The listing builds one solid part. Answer for the finished solid, in the listing's coordinates (mm). Coordinates: 2 decimals unless noted, no trailing zeros. Write each loop counter-clockwise with the first axis right and the second up, starting at its lowest first coordinate (ties: lowest second). Pieces come first, ordered by that corner, then holes.
from build123d import *

# Parameters (mm, degrees)
F2_SIZE2 = 0.21996
F2_SIZE  = 0.12699


# Not quite as in the source:
# - a fillet or chamfer is up to 0.001 mm smaller than in the source, because OpenCascade refuses the exact size


with BuildPart() as f1:
    # F0 (on Front) → F1 (revolve)
    with BuildSketch(Plane.XZ):
        Polygon((-38.1, 9.779), (0, 9.779), (0, 10.033), (-3.81, 10.033), (-3.81, 10.795), (-38.1, 10.795), align=None)
    revolve(axis=Axis((-19.05, 0, 0), (-1, 0, 0)))

    # F2 (size 0.127 and 0.2199704526 in the source; OpenCascade refuses exactly that, so slightly less here)
    f2_edges = [f1.edges().sort_by_distance(p)[0] for p in [
        (0, 0, -10.033),
        (0, 0, -9.779),
    ]]
    f2_side = f1.faces().sort_by_distance((0, 0, -9.807378))[0]
    chamfer(f2_edges, length=F2_SIZE, length2=F2_SIZE2, reference=f2_side)


solid = f1.part
Q1. Find the intervals of material crossed by probe 1 along Y at (x, z) = (-7.5, 0) (3 decimals); probe 2 along Z at (x, y) = (-5, -1); probe 3 along Z at (x, y) = (-15, 5), in increasing order.
Answers below:
probe 1: y = -10.795 to -9.779, 9.779 to 10.795
probe 2: z = -10.75 to -9.73, 9.73 to 10.75
probe 3: z = -9.57 to -8.4, 8.4 to 9.57
Q2. The part is cut by section C-C, the plane x = -11. Write down the section's boundary in (y, z) (3 decimals), then the cut area to 3 significant figures.
Answers below:
outline: circle Ø21.59 at (0, 0); hole circle Ø19.558 at (0, 0)
area: 65.7 mm2
Q3. Given pin 1 (1.5 mm diameter, centred on x = -33, z = 7, fed in from +Y); pin 2 (11 mm diameter, centred on y = 4, z = -3.5, fed in from +X); pin 3 (1.5 mm diameter, centred on x = -25, z = -2.5, fed in from -Y); pin 4 (3 mm diameter, centred on x = -19.5, y = 7, fed in from -Z), each flat-ended and moving along its own axis, determine where each tip first touches the part or whether it passes through.
Answers below:
pin 1: stops at y = 8.8
pin 2: stops at x = 0
pin 3: stops at y = -10.65
pin 4: stops at z = -9.29
Q4. Determine the mould class of faces 1 (the face through (-18.895, -9.546, -2.12)), 2 (the face through (-3.81, -10, -3)), 3 (the face through (-2.04, -9.794, -2.175)) for opening direction Z: released by +Z, released by -Z, zero draft, split by the parting line, or undercut.
Answers below:
face 1: undercut
face 2: zero draft
face 3: split by the parting line
